from build123d import *

# Parameters (mm, degrees)
CROQUIS1_W                   = 10
CROQUIS1_H                   = 10
SALIENTE_EXTRUIR1_DEPTH      = 37.5
TALADRO_DE_MARGEN_PARA_M33_D = 3.75
TALADRO_DE_MARGEN_PARA_M34_D = 3.75
CORTAR_EXTRUIR4_DEPTH        = 3.2
CORTAR_EXTRUIR5_DEPTH        = 3.2


with BuildPart() as part:
    # Croquis1 → Saliente-Extruir1 (new body, symmetric)
    with BuildSketch(Plane.XY):
        Rectangle(CROQUIS1_W, CROQUIS1_H)
    extrude(amount=SALIENTE_EXTRUIR1_DEPTH, both=True)

    # Taladro de margen para M33 (through all)
    with Locations(Plane.ZY.offset(5)):
        with Locations((-10, 0), (10, 0)):
            Hole(TALADRO_DE_MARGEN_PARA_M33_D / 2)

    # Taladro de margen para M34 (through all)
    with Locations(Plane(origin=(0, -5, 0), x_dir=(-1, 0, 0), z_dir=(0, -1, 0))):
        with Locations((0, 30), (0, -30)):
            Hole(TALADRO_DE_MARGEN_PARA_M34_D / 2)

    # Croquis19 → Cortar-Extruir4 (cut)
    with BuildSketch(Plane.XZ.offset(5)):
        Polygon((2.771281292, -28.4), (0, -26.8), (-2.771281292, -28.4), (-2.771281292, -31.6), (0, -33.2), (2.771281292, -31.6), align=None)
        Polygon((2.771281292, 31.6), (0, 33.2), (-2.771281292, 31.6), (-2.771281292, 28.4), (0, 26.8), (2.771281292, 28.4), align=None)
    extrude(amount=-CORTAR_EXTRUIR4_DEPTH, mode=Mode.SUBTRACT)

    # Croquis20 → Cortar-Extruir5 (cut)
    with BuildSketch(Plane.ZY.offset(5)):
        Polygon((-8.4, -2.771281292), (-6.8, 0), (-8.4, 2.771281292), (-11.6, 2.771281292), (-13.2, 0), (-11.6, -2.771281292), align=None)
        Polygon((11.6, -2.771281292), (13.2, 0), (11.6, 2.771281292), (8.4, 2.771281292), (6.8, 0), (8.4, -2.771281292), align=None)
    extrude(amount=-CORTAR_EXTRUIR5_DEPTH, mode=Mode.SUBTRACT)


solid = part.part
Read the model definition and answer for the solid it produces. Units are mm, in the model's axes. A direction names the side the tool comes from. Give positions to 0.01 mm unless a question says otherwise; leave off trailing zeros. Write each loop counter-clockwise with the first axis right and the second up, starting at its lowest first coordinate (ties: lowest second). Pieces come first, ordered by that corner, then holes. Notation, with made-up numbers: M 63,71 L 103,71 A30 ccw 103,101 Z; hole C 15,-13 d10. An arc over 180 degrees is marked long. One line per item, written item: value. Start each with the question number.
(1) Determine the mould class of faces 1 (the flat face through (-3.42, 1.37, -7.59)), 2 (the flat face through (-1.405, -3.422, 27.611)), 3 (the flat face through (-5, 0, 1)) for opening direction X: pulls with the +X half, pulls with the -X half, needs draft (parallel to the pull), parting line crosses it, or undercut.
(2) Find section A-A (z = -10). Determine the outline of the cut face in (x, y) (3 decimals), plus the area to 3 significant figures.
(3) Find the intervals of material crossed by line 1 (Z direction, x = 0, y = 2) (3 decimals); line 2 (Z direction, x = 1, y = -0.75); line 3 (Z direction, x = 0.5, y = -3), in increasing order.
(4) Find section B-B (y = -4.25). Determine the outline of the cut face in (x, z).
(5) Find section D-D (y = 1.25). Determine the outline of the cut face in (x, z) (3 decimals), plus the area to 3 significant figures.
(6) Find section C-C (x = 1). Determine the outline of the cut face in (y, z) (3 decimals).
(7) A tool of negligible diameter and unlimited length cuts with its end or side. For faces 4 (the flat face through (0, 5, 1)), 5 (the flat face through (-3.422, -1.405, -7.611)), 6 (the flat face through (1.405, -3.422, -27.611)), from which of +Z, -Z, +X, -X, +Y, -Y can it reach the whole face along a straight path? Write none if from no direction.
Results below:
1. face 1: needs draft
1. face 2: undercut
1. face 3: pulls with the -X half
2. outline: M -5,-5 L 5,-5 L 5,-1.875 L -1.8,-1.875 L -1.8,-2.771 L -5,-2.771 Z; M -5,2.771 L -1.8,2.771 L -1.8,1.875 L 5,1.875 L 5,5 L -5,5 Z
2. area: 56.8 mm^2
3. line 1: z = -37.5 to -31.875, -28.125 to 28.125, 31.875 to 37.5
3. line 2: z = -37.5 to -31.59, -28.41 to -11.72, -8.28 to 8.28, 11.72 to 28.41, 31.59 to 37.5
3. line 3: z = -37.5 to -32.91, -27.09 to 27.09, 32.91 to 37.5
4. outline: M -5,-37.5 L 5,-37.5 L 5,37.5 L -5,37.5 Z; hole M -2.77,-31.6 L 0,-33.2 L 2.77,-31.6 L 2.77,-28.4 L 0,-26.8 L -2.77,-28.4 Z; hole M -2.77,28.4 L 0,26.8 L 2.77,28.4 L 2.77,31.6 L 0,33.2 L -2.77,31.6 Z
5. outline: M -5,-37.5 L 5,-37.5 L 5,-11.398 L -1.8,-11.398 L -1.8,-12.478 L -5,-12.478 Z; M -5,-7.522 L -1.8,-7.522 L -1.8,-8.602 L 5,-8.602 L 5,8.602 L -1.8,8.602 L -1.8,7.522 L -5,7.522 Z; M -5,12.478 L -1.8,12.478 L -1.8,11.398 L 5,11.398 L 5,37.5 L -5,37.5 Z; hole C 0,-30 d3.75; hole C 0,30 d3.75
5. area: 658 mm^2
6. outline: M -5,-37.5 L 5,-37.5 L 5,-31.586 L -1.8,-31.586 L -1.8,-32.623 L -5,-32.623 Z; M -5,-27.377 L -1.8,-27.377 L -1.8,-28.414 L 5,-28.414 L 5,28.414 L -1.8,28.414 L -1.8,27.377 L -5,27.377 Z; M -5,32.623 L -1.8,32.623 L -1.8,31.586 L 5,31.586 L 5,37.5 L -5,37.5 Z; hole C 0,-10 d3.75; hole C 0,10 d3.75
7. face 4: +Z, -Z, +X, -X, +Y
7. face 5: -X
7. face 6: -Y
